Source: CAD feature listing. Evaluate the final solid. Frame: model axes, mm. A direction names the side the tool comes from. Round coordinates to 2 decimals unless told otherwise and drop trailing zeros. Loops run counter-clockwise (first coordinate to the right, second up) from the corner with the lowest first, then second, coordinate; pieces in that order, holes last. Notation, with made-up numbers: (72.25, 85.25) - (117.25, 85.25) arc R26 cw to (117.25, 123.25) - close; hole circle Ø2 at (-33.5, 9.5). An arc over 180 degrees is marked (long way). One line per question, with ' | ' between items. Start each with the question number.
1. Cut plane A-A (y = -10). Return loops of the section in (x, z).
2. Cut plane B-B (y = -77). Return loops of the section in (x, z), then the cut area to 3 significant figures.
3. Mould query, pull axis Z, two halves, no side actions, for faces 3 (the conical face through (-0.41, -17.777, -0.17)), 4 (the cylindrical face through (-5.506, -46.958, -24.796)), 5 (the flat face through (0, -101.6, 0)). Classes: pulls with the +Z half, pulls with the -Z half, needs draft (parallel to the pull), parting line crosses it, or undercut.
4. Access query for faces 1 (the cylindrical face through (2.435, -8.371, 0.767)), 2 (the flat face through (5, 0, 0)). Directions: +Z, -Z, +X, -X, +Y, -Y. A direction counts if a zero-diameter tool reaches every point of the face in a straight line with its end or side. Return the directions, or none.
5. Ray query, line 1 (Z direction, x = 0, y = -7); line 2 (X direction, y = -90, z = -4); line 3 (Y direction, x = -8.5, z = -17.5). Return the intervals inside material, ascending.
6. Pin query (flat end, axial travel): pin 1 (8 mm diameter, centred on y = -90.5, z = 16.5, fed in from +X); pin 2 (8 mm diameter, centred on x = 8.5, y = -62, fed in from -Z); pin 3 (3 mm diameter, centred on x = -4, y = -61, fed in from +Z). Return the tip coordinate at first contact, or that it passes through.
```python
from build123d import *

# Parameters (mm, degrees)
F0_R     = 25.4
F1_DEPTH = 101.6
F2_R     = 6.35
F4_D     = 5.1054
F4_DEPTH = 16.51
F4_TIP   = 1.5338169022


with BuildPart() as f1:
    # F0 (on Front) → F1 (new body)
    with BuildSketch(Plane.XZ):
        Circle(F0_R)
    extrude(amount=F1_DEPTH)

    # F2
    f2_edges = [f1.edges().sort_by_distance(p)[0] for p in [
        (-25.4, -101.6, 0),
    ]]
    fillet(f2_edges, radius=F2_R)

    # F4
    with Locations(Plane(origin=(0, 0, 0), x_dir=(-1, 0, 0), z_dir=(0, 1, 0))):
        with Locations((0, 0)):
            Hole(F4_D / 2, depth=F4_DEPTH)
            with Locations((0, 0, -(F4_DEPTH + F4_TIP / 2))):  # 118° drill point
                Cone(0, F4_D / 2, F4_TIP, mode=Mode.SUBTRACT)


solid = f1.part
```
Answers follow:
1) outline: circle Ø50.8 at (0, 0); hole circle Ø5.11 at (0, 0)
2) outline: circle Ø50.8 at (0, 0) | area: 2,030 mm2
3) face 3: undercut | face 4: parting line crosses it | face 5: needs draft
4) face 1: +Y | face 2: +Z, -Z, +X, -X, +Y
5) line 1: z = -25.4 to -2.55, 2.55 to 25.4 | line 2: x = -25.08 to 25.08 | line 3: y = -101.59 to 0
6) pin 1: stops at x = 22.11 | pin 2: stops at z = -25 | pin 3: stops at z = 25.28
